```python
from build123d import *

# Parameters (mm, degrees)
F0_W      = 20
F0_H      = 10
F1_DEPTH  = 30
F1_FACE_W = 20
F1_FACE_H = 10
F2_DEPTH  = 10
F4_R      = 5
F5_DEPTH  = 8


with BuildPart() as f1:
    # F0 (on Front) → F1 (new body)
    with BuildSketch(Plane.XZ):
        with Locations((0, 5)):
            Rectangle(F0_W, F0_H)
    extrude(amount=F1_DEPTH)

    # F1_face (on face) → F2 (join)
    with BuildSketch(Plane(origin=(0, 0, 5), x_dir=(1, 0, 0), z_dir=(0, 1, 0))):
        Rectangle(F1_FACE_W, F1_FACE_H)
    extrude(amount=F2_DEPTH)

    # F4 (on face) → F5 (cut)
    with BuildSketch(Plane.XY.offset(10)):
        Circle(F4_R)
    extrude(amount=-F5_DEPTH, mode=Mode.SUBTRACT)


solid = f1.part
```
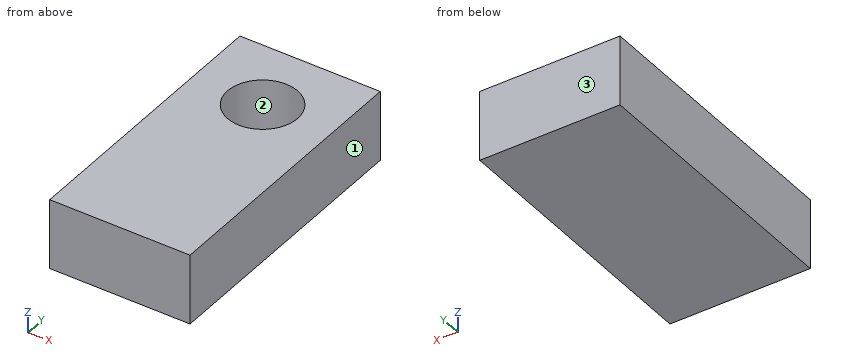
Build history of the part. All positions in model axes, mm. Face numbers are marked on the shaded views. Give positions to 0.01 mm unless a question says otherwise; leave off trailing zeros. Loops run counter-clockwise (first coordinate to the right, second up) from the corner with the lowest first, then second, coordinate; pieces in that order, holes last.
1) Drop a flat-ended pin along its axis: P1, Ø3, axis at x = 2.5, y = 1.5, coming from the +Z side. Give the stop position or say it passes through.
Values follow:
P1: stops at z = 2
2) Band-saw the part on B-B on x = 0. List the corners of the cut face in (y, z), then the cut area to 3 significant figures.
Values follow:
outline: (-30, 0) - (10, 0) - (10, 10) - (5, 10) - (5, 2) - (-5, 2) - (-5, 10) - (-30, 10) - close
area: 320 mm2
3) Band-saw the part on A-A on y = 4. List the corners of the cut face in (x, z), then the cut area to 3 significant figures.
Values follow:
outline: (-10, 0) - (10, 0) - (10, 10) - (3, 10) - (3, 2) - (-3, 2) - (-3, 10) - (-10, 10) - close
area: 152 mm2
4) Band-saw the part on C-C on z = 7.25. List the corners of the cut face in (x, y).
Values follow:
outline: (-10, -30) - (10, -30) - (10, 10) - (-10, 10) - close; hole circle Ø10 at (0, 0)
5) Probe line 1 along Y through (x, z) = (0, 7); line 2 along X through (y, z) = (-4, 5); line 3 along X through (y, z) = (-2, 5.25). List the from-to ranges inside material, lowest first.
Values follow:
line 1: y = -30 to -5, 5 to 10
line 2: x = -10 to -3, 3 to 10
line 3: x = -10 to -4.58, 4.58 to 10
6) Two-plate mould, pull along Y, no slides. Class the marked faces 1, 2 and 3: released by +Y, released by -Y, zero draft, split by the parting line, or undercut.
Values follow:
face 1: zero draft
face 2: undercut
face 3: released by +Y
